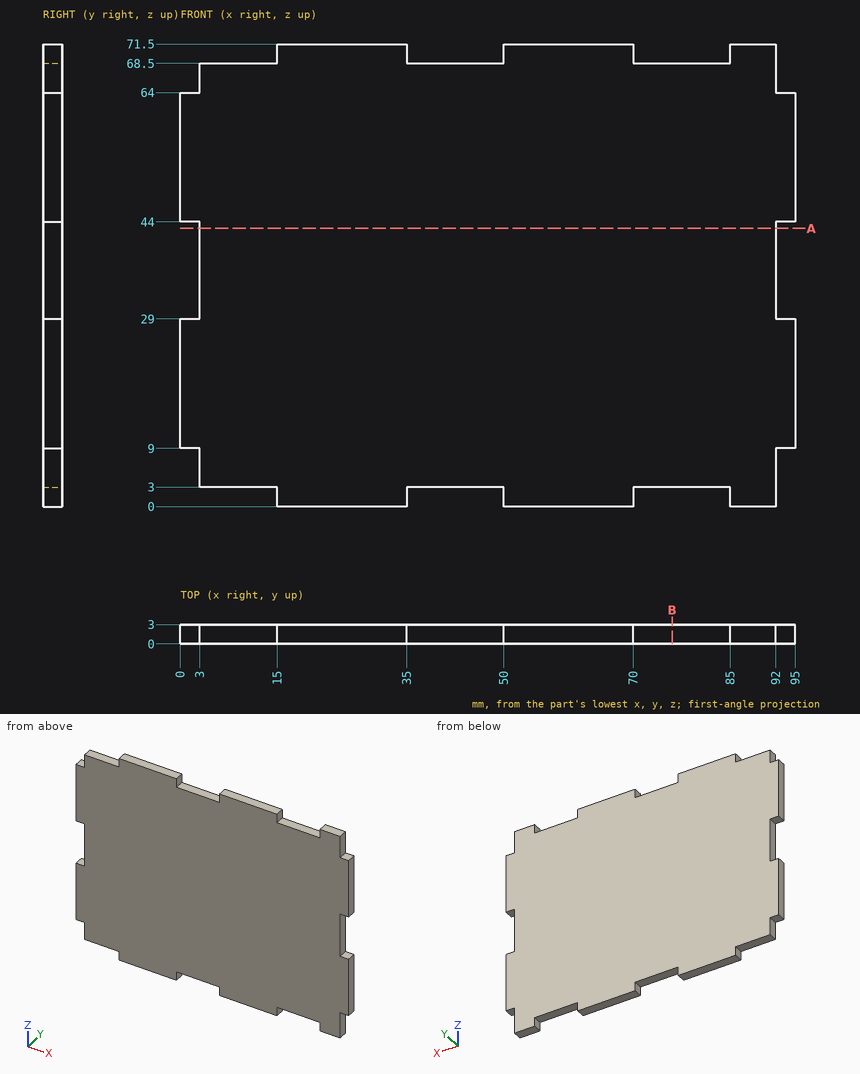
The figure shows three views and two pictorial views of one solid part (mm, origin at its lowest corner). Answer the questions. Round coordinates to 2 decimals unless told otherwise and drop trailing zeros. Order: outer loops, then holes, each group sorted by start corner. A loop starts at its lowest first (then second) coordinate and runs counter-clockwise, first axis right, second up. Notation, with made-up numbers: M -12.75,42 L 12.25,42 A22 cw 12.25,62 Z; hole C -4,64.5 d10. An arc over 180 degrees is marked long. Put each result on its own line as item: value. Start each with the question number.
Q1. Straight lines are drawn through the part: L1, parallel to Z at x = 36, y = 1.3; L2, parallel to X at y = 1.6, z = 42.5. For each, find the intervals that lie inside material, in ascending order. Write a range as [from, to].
Q2. Section A-A, the plane z = 43 is taken. Write down the section's boundary in (x, y).
Q3. Flat-ended cylindrical pins translate along their axes: pin 1 (0.9 mm diameter, centred on y = 2, z = 69.5, fed in from +X); pin 2 (5 mm diameter, centred on x = 75.5, z = 17, fed in from -Y); pin 3 (0.9 mm diameter, centred on x = 93, y = 2, fed in from +Z). Find the tip coordinate at first contact, or state that the pin passes through.
Q4. Section B-B, the plane x = 76 is taken. Write down the section's boundary in (y, z).
Findings below:
1. L1: z = [3, 68.5]
1. L2: x = [3, 92]
2. outline: M 3,0 L 92,0 L 92,3 L 3,3 Z
3. pin 1: stops at x = 92
3. pin 2: stops at y = 0
3. pin 3: stops at z = 64
4. outline: M 0,3 L 3,3 L 3,68.5 L 0,68.5 Z
